Work out the finished part from the listing and answer in its coordinate system (mm). A direction names the side the tool comes from. Give positions to 0.01 mm unless a question says otherwise; leave off trailing zeros. Order: outer loops, then holes, each group sorted by start corner. A loop starts at its lowest first (then second) coordinate and runs counter-clockwise, first axis right, second up. Notation, with made-up numbers: (0.25, 19.5) - (23.25, 19.5) arc R14 ccw to (23.25, 46.5) - close; hole circle Ø7 at (17, 20). An arc over 180 degrees is marked (long way). Return JSON: item names as keys, results as strings. Group by question number.
from build123d import *
from OCP.BRepFilletAPI import BRepFilletAPI_MakeChamfer

# Parameters (mm, degrees)
SKETCH1_W                                  = 119.52
SKETCH1_H                                  = 86.5
BOSS_EXTRUDE1_DEPTH                        = 88.24
SHELL1_T                                   = -5
CHAMFER1_SIZE                              = 2.5
CHAMFER1_SIZE2                             = 2.979383981
CHAMFER2_SIZE                              = 2.5
CHAMFER2_SIZE2                             = 2.979383981
CHAMFER3_SIZE                              = 2.5
CHAMFER3_SIZE2                             = 2.979383981
CUT_EXTRUDE1_REACH                         = 156.732
SKETCH3_W                                  = 70
SKETCH3_H                                  = 66.5
FILLET1_R                                  = 2
FILLET1_OF_MIRROR1_R                       = 2
SKETCH4_W                                  = 109.52
SKETCH4_H                                  = 5
BOSS_EXTRUDE2_DEPTH                        = 5
CUT_EXTRUDE2_REACH                         = 139.258
SKETCH5_R                                  = 0.95
BOSS_EXTRUDE3_DEPTH                        = 8.5
BOSS_EXTRUDE4_DEPTH                        = 5
BOSS_EXTRUDE6_DEPTH                        = 35
BOSS_EXTRUDE7_DEPTH                        = 8.5
BOSS_EXTRUDE8_DEPTH                        = 35
BOSS_EXTRUDE9_DEPTH                        = 38.5
SKETCH16_W                                 = 5
SKETCH16_H                                 = 27.5
BOSS_EXTRUDE10_DEPTH                       = 3
MIRROR7_COPY_1_SKETCH_W                    = 5
MIRROR7_COPY_1_SKETCH_H                    = 27.5
MIRROR7_COPY_1_DEPTH                       = 3
SKETCH15_R                                 = 1.45
CUT_EXTRUDE5_DEPTH                         = 8
MIRROR8_AT_THE_SECOND_PLANE_COPY_1_SKETC_R = 1.45
MIRROR8_AT_THE_SECOND_PLANE_COPY_1_DEPTH   = 8
SKETCH17_R                                 = 1.45
CUT_EXTRUDE6_DEPTH                         = 8
SKETCH18_R                                 = 1.45
CUT_EXTRUDE7_DEPTH                         = 8
SKETCH19_W                                 = 15
SKETCH19_H                                 = 15
CUT_EXTRUDE8_DEPTH                         = 5
FILLET2_R                                  = 1
FILLET2_OF_MIRROR10_R                      = 1


with BuildPart() as part:
    # Sketch1 → Boss-Extrude1 (new body)
    with BuildSketch(Plane.XY):
        Rectangle(SKETCH1_W, SKETCH1_H)
    extrude(amount=BOSS_EXTRUDE1_DEPTH)

    # Shell1
    shell1_openings = [part.faces().sort_by_distance(p)[0] for p in [
        (0, 0, 0),
    ]]
    offset(amount=SHELL1_T, openings=shell1_openings, kind=Kind.INTERSECTION)

    # Chamfer1: one chamfer whose edges measure the first distance from different faces: ONE call of the kernel's chamfer builder (chamfer() names one face for all edges)
    chamfer1_edges_1 = [part.edges().sort_by_distance(p)[0] for p in [
        (59.76, 0, 88.24),
    ]]
    chamfer1_side_1 = [part.faces().sort_by_distance(p)[0] for p in [
        (59.76, 0, 44.12),
    ]]
    chamfer1_edges_2 = [part.edges().sort_by_distance(p)[0] for p in [
        (0, 43.25, 88.24),
    ]]
    chamfer1_side_2 = [part.faces().sort_by_distance(p)[0] for p in [
        (0, 43.25, 44.12),
    ]]
    chamfer1_edges_3 = [part.edges().sort_by_distance(p)[0] for p in [
        (-59.76, 0, 88.24),
    ]]
    chamfer1_side_3 = [part.faces().sort_by_distance(p)[0] for p in [
        (-59.76, 0, 44.12),
    ]]
    chamfer1_edges_4 = [part.edges().sort_by_distance(p)[0] for p in [
        (0, -43.25, 88.24),
    ]]
    chamfer1_side_4 = [part.faces().sort_by_distance(p)[0] for p in [
        (0, -43.25, 44.12),
    ]]
    chamfer1 = BRepFilletAPI_MakeChamfer(part.part.solid().wrapped)
    for e in chamfer1_edges_1:
        chamfer1.Add(CHAMFER1_SIZE, CHAMFER1_SIZE2, e.wrapped, chamfer1_side_1[0].wrapped)  # the first distance lies on this face
    for e in chamfer1_edges_2:
        chamfer1.Add(CHAMFER1_SIZE, CHAMFER1_SIZE2, e.wrapped, chamfer1_side_2[0].wrapped)  # the first distance lies on this face
    for e in chamfer1_edges_3:
        chamfer1.Add(CHAMFER1_SIZE, CHAMFER1_SIZE2, e.wrapped, chamfer1_side_3[0].wrapped)  # the first distance lies on this face
    for e in chamfer1_edges_4:
        chamfer1.Add(CHAMFER1_SIZE, CHAMFER1_SIZE2, e.wrapped, chamfer1_side_4[0].wrapped)  # the first distance lies on this face
    add(Compound.cast(chamfer1.Shape()), mode=Mode.REPLACE)

    # Chamfer2
    chamfer2_edges = [part.edges().sort_by_distance(p)[0] for p in [
        (-59.76, 43.25, 42.87),
    ]]
    chamfer2_side = [part.faces().sort_by_distance(p)[0] for p in [
        (0, 43.25, 42.87),
    ]]
    chamfer(chamfer2_edges, length=CHAMFER2_SIZE, length2=CHAMFER2_SIZE2, reference=chamfer2_side[0])

    # Chamfer3: one chamfer whose edges measure the first distance from different faces: ONE call of the kernel's chamfer builder (chamfer() names one face for all edges)
    chamfer3_edges_1 = [part.edges().sort_by_distance(p)[0] for p in [
        (59.76, -43.25, 42.87),
    ]]
    chamfer3_side_1 = [part.faces().sort_by_distance(p)[0] for p in [
        (0, -43.25, 42.87),
    ]]
    chamfer3_edges_2 = [part.edges().sort_by_distance(p)[0] for p in [
        (-59.76, -43.25, 42.87),
    ]]
    chamfer3_side_2 = [part.faces().sort_by_distance(p)[0] for p in [
        (-59.76, -1.489691991, 42.87),
    ]]
    chamfer3_edges_3 = [part.edges().sort_by_distance(p)[0] for p in [
        (59.76, 43.25, 42.87),
    ]]
    chamfer3_side_3 = [part.faces().sort_by_distance(p)[0] for p in [
        (59.76, 0, 42.87),
    ]]
    chamfer3 = BRepFilletAPI_MakeChamfer(part.part.solid().wrapped)
    for e in chamfer3_edges_1:
        chamfer3.Add(CHAMFER3_SIZE, CHAMFER3_SIZE2, e.wrapped, chamfer3_side_1[0].wrapped)  # the first distance lies on this face
    for e in chamfer3_edges_2:
        chamfer3.Add(CHAMFER3_SIZE, CHAMFER3_SIZE2, e.wrapped, chamfer3_side_2[0].wrapped)  # the first distance lies on this face
    for e in chamfer3_edges_3:
        chamfer3.Add(CHAMFER3_SIZE, CHAMFER3_SIZE2, e.wrapped, chamfer3_side_3[0].wrapped)  # the first distance lies on this face
    add(Compound.cast(chamfer3.Shape()), mode=Mode.REPLACE)

    # Sketch3 → Cut-Extrude1 (cut, up to next)
    with BuildSketch(Plane(origin=(59.76, 0, 0), x_dir=(0, 0, -1), z_dir=(1, 0, 0)), mode=Mode.PRIVATE) as cut_extrude1_sk1:
        with Locations((-35, 0)):
            Rectangle(SKETCH3_W, SKETCH3_H)
    cut_extrude1_tool1 = extrude(cut_extrude1_sk1.sketch, amount=-CUT_EXTRUDE1_REACH, mode=Mode.PRIVATE) & part.part
    cut_extrude1 = cut_extrude1_tool1.solids().sort_by_distance((59.76, 0, 35))[0]
    add(cut_extrude1, mode=Mode.SUBTRACT)

    # Fillet1
    fillet1_edges = [part.edges().sort_by_distance(p)[0] for p in [
        (57.26, -33.25, 70),
        (57.26, 33.25, 70),
    ]]
    fillet(fillet1_edges, radius=FILLET1_R)

    # Mirror1: Cut-Extrude1 across plane
    add(cut_extrude1.mirror(Plane(origin=(0, 0, 0), x_dir=(0, 0, 1), z_dir=(1, 0, 0))), mode=Mode.SUBTRACT)

    # Fillet1 of Mirror1
    fillet1_of_mirror1_edges = [part.edges().sort_by_distance(p)[0] for p in [
        (-57.26, -33.25, 70),
        (-57.26, 33.25, 70),
    ]]
    fillet(fillet1_of_mirror1_edges, radius=FILLET1_OF_MIRROR1_R)

    # Sketch4 → Boss-Extrude2 (add)
    with BuildSketch(Plane(origin=(0, 0, 0), x_dir=(-1, 0, 0), z_dir=(0, 0, -1))):
        with Locations((0, 40.75)):
            Rectangle(SKETCH4_W, SKETCH4_H)
    extrude(amount=BOSS_EXTRUDE2_DEPTH)

    # Sketch5 → Cut-Extrude2 (cut, up to next)
    with BuildSketch(Plane(origin=(0, 43.25, 0), x_dir=(1, 0, 0), z_dir=(0, 1, 0)), mode=Mode.PRIVATE) as cut_extrude2_sk1:
        with Locations(Location((-52.76, 2.5, 0), (0, 0, 270))):
            Circle(SKETCH5_R)
    cut_extrude2_tool1 = extrude(cut_extrude2_sk1.sketch, amount=-CUT_EXTRUDE2_REACH, mode=Mode.PRIVATE) & part.part
    # Sketch5 → Cut-Extrude2 (cut, up to next)
    with BuildSketch(Plane(origin=(0, 43.25, 0), x_dir=(1, 0, 0), z_dir=(0, 1, 0)), mode=Mode.PRIVATE) as cut_extrude2_sk2:
        with Locations(Location((52.76, 2.5, 0), (0, 0, 270))):
            Circle(SKETCH5_R)
    cut_extrude2_tool2 = extrude(cut_extrude2_sk2.sketch, amount=-CUT_EXTRUDE2_REACH, mode=Mode.PRIVATE) & part.part
    add(cut_extrude2_tool1.solids().sort_by_distance((-52.76, 43.25, -2.5))[0], mode=Mode.SUBTRACT)
    add(cut_extrude2_tool2.solids().sort_by_distance((52.76, 43.25, -2.5))[0], mode=Mode.SUBTRACT)

    # Sketch6 → Boss-Extrude3 (add)
    with BuildSketch(Plane(origin=(0, 0, 0), x_dir=(-1, 0, 0), z_dir=(0, 0, -1))):
        Polygon((-59.76, -33.25), (-54.86, -33.25), (-54.86, -43.25), (-57.26, -43.25), (-59.76, -40.270616019), align=None)
    extrude(amount=BOSS_EXTRUDE3_DEPTH)

    # Sketch8 → Boss-Extrude4 (add)
    with BuildSketch(Plane(origin=(0, 0, 0), x_dir=(-1, 0, 0), z_dir=(0, 0, -1))):
        Polygon((57.26, 43.25), (54.76, 43.25), (54.76, 38.25), (54.76, 33.25), (59.76, 33.25), (59.76, 40.270616019), align=None)
        Polygon((-54.76, 33.25), (-54.76, 38.25), (-54.76, 43.25), (-56.780616019, 43.25), (-59.76, 40.75), (-59.76, 33.25), align=None)
    extrude(amount=BOSS_EXTRUDE4_DEPTH)

    # Sketch10 → Boss-Extrude6 (add)
    with BuildSketch(Plane(origin=(0, 0, -5), x_dir=(-1, 0, 0), z_dir=(0, 0, -1))):
        Polygon((-59.76, 40.75), (-59.76, 43.25), (-56.780616019, 43.25), align=None)
    extrude(amount=-BOSS_EXTRUDE6_DEPTH)

    # Sketch11 → Boss-Extrude7 (add)
    with BuildSketch(Plane(origin=(0, 0, 0), x_dir=(-1, 0, 0), z_dir=(0, 0, -1))):
        Polygon((59.76, -33.25), (54.86, -33.25), (54.86, -43.25), (56.780616019, -43.25), (59.76, -40.75), align=None)
    extrude(amount=BOSS_EXTRUDE7_DEPTH)

    # Sketch13 → Boss-Extrude8 (add)
    with BuildSketch(Plane(origin=(0, 0, -5), x_dir=(-1, 0, 0), z_dir=(0, 0, -1))):
        Polygon((57.26, 43.25), (59.76, 43.25), (59.76, 40.270616019), align=None)
    extrude(amount=-BOSS_EXTRUDE8_DEPTH)

    # Sketch14 → Boss-Extrude9 (add)
    with BuildSketch(Plane(origin=(0, 0, -8.5), x_dir=(-1, 0, 0), z_dir=(0, 0, -1))):
        Polygon((-59.76, -40.270616019), (-59.76, -43.25), (-57.26, -43.25), align=None)
        Polygon((59.76, -40.75), (59.76, -43.25), (56.780616019, -43.25), align=None)
    extrude(amount=-BOSS_EXTRUDE9_DEPTH)

    # Sketch16 → Boss-Extrude10 (add)
    with BuildSketch(Plane.XZ.offset(-38.25)):
        with Locations((52.26, 16.25)):
            Rectangle(SKETCH16_W, SKETCH16_H)
    boss_extrude10 = extrude(amount=BOSS_EXTRUDE10_DEPTH)

    # Mirror6: Boss-Extrude10 across plane
    add(boss_extrude10.mirror(Plane(origin=(0, 0, 0), x_dir=(0, 0, 1), z_dir=(1, 0, 0))))

    # Mirror7: Boss-Extrude10 across plane
    add(boss_extrude10.mirror(Plane.ZX))

    # Mirror7 copy 1 sketch → Mirror7 copy 1 (add)
    with BuildSketch(Plane(origin=(0, -38.25, 0), x_dir=(-1, 0, 0), z_dir=(0, 1, 0))):
        with Locations((52.26, 16.25)):
            Rectangle(MIRROR7_COPY_1_SKETCH_W, MIRROR7_COPY_1_SKETCH_H)
    extrude(amount=MIRROR7_COPY_1_DEPTH)

    # Sketch15 → Cut-Extrude5 (cut)
    with BuildSketch(Plane(origin=(59.76, 0, 0), x_dir=(0, 0, -1), z_dir=(1, 0, 0))):
        with Locations((-6.4, 37.5)):
            Circle(SKETCH15_R)
        with Locations((-23.4, 37.5)):
            Circle(SKETCH15_R)
    cut_extrude5 = extrude(amount=-CUT_EXTRUDE5_DEPTH, mode=Mode.SUBTRACT)

    # Mirror8: Cut-Extrude5 across plane
    add(cut_extrude5.mirror(Plane.ZX), mode=Mode.SUBTRACT)

    # Mirror8 at the second plane: Cut-Extrude5 across plane
    add(cut_extrude5.mirror(Plane(origin=(0, 0, 0), x_dir=(0, 0, 1), z_dir=(1, 0, 0))), mode=Mode.SUBTRACT)

    # Mirror8 at the second plane copy 1 sketc → Mirror8 at the second plane copy 1 (cut)
    with BuildSketch(Plane(origin=(-59.76, 0, 0), x_dir=(0, 0, -1), z_dir=(-1, 0, 0))):
        with Locations((-6.4, 37.5)):
            Circle(MIRROR8_AT_THE_SECOND_PLANE_COPY_1_SKETC_R)
        with Locations((-23.4, 37.5)):
            Circle(MIRROR8_AT_THE_SECOND_PLANE_COPY_1_SKETC_R)
    extrude(amount=-MIRROR8_AT_THE_SECOND_PLANE_COPY_1_DEPTH, mode=Mode.SUBTRACT)

    # Sketch17 → Cut-Extrude6 (cut)
    with BuildSketch(Plane(origin=(59.76, 0, 0), x_dir=(0, 0, -1), z_dir=(1, 0, 0))):
        with Locations((5.5, -37.5)):
            Circle(SKETCH17_R)
    extrude(amount=-CUT_EXTRUDE6_DEPTH, mode=Mode.SUBTRACT)

    # Sketch18 → Cut-Extrude7 (cut)
    with BuildSketch(Plane(origin=(-54.86, 0, 0), x_dir=(0, 0, -1), z_dir=(1, 0, 0))):
        with Locations((5.5, -37.5)):
            Circle(SKETCH18_R)
    extrude(amount=-CUT_EXTRUDE7_DEPTH, mode=Mode.SUBTRACT)

    # Sketch19 → Cut-Extrude8 (cut)
    with BuildSketch(Plane(origin=(0, 43.25, 0), x_dir=(1, 0, 0), z_dir=(0, 1, 0))):
        with Locations((-37.26, -14.5)):
            Rectangle(SKETCH19_W, SKETCH19_H)
    cut_extrude8 = extrude(amount=-CUT_EXTRUDE8_DEPTH, mode=Mode.SUBTRACT)

    # Fillet2
    fillet2_edges = [part.edges().sort_by_distance(p)[0] for p in [
        (-44.76, 40.75, 22),
        (-44.76, 40.75, 7),
        (-29.76, 40.75, 7),
        (-29.76, 40.75, 22),
    ]]
    fillet(fillet2_edges, radius=FILLET2_R)

    # Mirror10: Cut-Extrude8 across plane
    add(cut_extrude8.mirror(Plane(origin=(0, 0, 0), x_dir=(0, 0, 1), z_dir=(1, 0, 0))), mode=Mode.SUBTRACT)

    # Fillet2 of Mirror10
    fillet2_of_mirror10_edges = [part.edges().sort_by_distance(p)[0] for p in [
        (44.76, 40.75, 22),
        (44.76, 40.75, 7),
        (29.76, 40.75, 7),
        (29.76, 40.75, 22),
    ]]
    fillet(fillet2_of_mirror10_edges, radius=FILLET2_OF_MIRROR10_R)


solid = part.part
1. The part is cut by section D-D (z = 26.5). Give the vertices of the cut face in (x, y), and give its area (3 significant figures).
2. The part is cut by section C-C (y = -15.5). Give the vertices of the cut face in (x, z), and give its area (3 significant figures).
3. A tool of negligible diameter and unlimited length cuts with its end or side. For faces 1 (the flat face through (-51.76, 38, 23)), 2 (the flat face through (51.76, 38, 23)), 3 (the flat face through (54.76, 0, 75)), from which of +Z, -Z, +X, -X, +Y, -Y can it reach the whole face along a straight path? Write none if from no direction.
4. The part is cut by section B-B (x = 37). Give the vertices of the cut face in (y, z).
5. Determine the mould class of faces 4 (the flat face through (-1, -38.25, 41)), 5 (the flat face through (-49.76, 37, 16)), 6 (the flat face through (-1, -40, 0)), 7 (the flat face through (-0.818, -41.739, 87.008)) for opening direction Y: released by +Y, released by -Y, zero draft, split by the parting line, or undercut.
6. The part is cut by section A-A (z = 41). Give the vertices of the cut face in (x, y).
7. Consider probe 1 along Y at (x, z) = (-57, 6.4); probe 2 along Y at (x, z) = (-53.5, 6.4); probe 3 along Y at (x, z) = (-0.5, 55.5). Determine where each line is inside the solid, lowest interval first. Write a range as from..to.
8. Each of these flat-tipped pins is pushed along its axis until it touches: pin 1 (1.5 mm diameter, centred on x = -51.5, y = 36.5, fed in from -Z); pin 2 (12 mm diameter, centred on y = -33, z = 64.5, fed in from +X); pin 3 (8 mm diameter, centred on x = 8.5, y = 32, fed in from -Z); pin 4 (0.8 mm diameter, centred on x = 58, y = 42, fed in from +Z). Where does it stop, or does it pass through?
Answers:
{
 "1": {"outline": "(-59.76, -43.25) - (59.76, -43.25) - (59.76, -33.25) - (54.76, -33.25) - (54.76, -35.25) - (49.76, -35.25) - (49.76, -38.25) - (-49.76, -38.25) - (-49.76, -35.25) - (-54.76, -35.25) - (-54.76, -33.25) - (-59.76, -33.25) - close; (-59.76, 33.25) - (-54.76, 33.25) - (-54.76, 35.25) - (-49.76, 35.25) - (-49.76, 38.25) - (49.76, 38.25) - (49.76, 35.25) - (54.76, 35.25) - (54.76, 33.25) - (59.76, 33.25) - (59.76, 43.25) - (-59.76, 43.25) - close", "area": "1,360 mm^2"},
 "2": {"outline": "(-59.76, 70) - (-54.76, 70) - (-54.76, 83.24) - (54.76, 83.24) - (54.76, 70) - (59.76, 70) - (59.76, 85.74) - (56.78, 88.24) - (-56.78, 88.24) - (-59.76, 85.74) - close", "area": "723 mm^2"},
 "3": {"face 1": "-X", "face 2": "+X", "face 3": "none"},
 "4": {"outline": "(-43.25, 0) - (-38.25, 0) - (-38.25, 83.24) - (38.25, 83.24) - (38.25, 22) - (43.25, 22) - (43.25, 85.74) - (40.27, 88.24) - (-40.27, 88.24) - (-43.25, 85.74) - close; (38.25, -5) - (43.25, -5) - (43.25, 7) - (38.25, 7) - close"},
 "5": {"face 4": "undercut", "face 5": "undercut", "face 6": "zero draft", "face 7": "released by -Y"},
 "6": {"outline": "(-59.76, -40.75) - (-56.78, -43.25) - (57.26, -43.25) - (59.76, -40.27) - (59.76, -33.25) - (54.76, -33.25) - (54.76, -38.25) - (-54.76, -38.25) - (-54.76, -33.25) - (-59.76, -33.25) - close; (-59.76, 33.25) - (-54.76, 33.25) - (-54.76, 38.25) - (54.76, 38.25) - (54.76, 33.25) - (59.76, 33.25) - (59.76, 40.75) - (56.78, 43.25) - (-57.26, 43.25) - (-59.76, 40.27) - close"},
 "7": {"probe 1": "y = -43.25..-38.95, -36.05..-33.25, 33.25..36.05, 38.95..43.25", "probe 2": "y = -43.25..-38.95, -36.05..-35.25, 35.25..36.05, 38.95..43.25", "probe 3": "y = -43.25..-38.25, 38.25..43.25"},
 "8": {"pin 1": "stops at z = 2.5", "pin 2": "stops at x = 59.76", "pin 3": "stops at z = 83.24", "pin 4": "stops at z = 87.12"}
}
